from build123d import *

# Parameters (mm, degrees)
F0_R      = 20
F1_DEPTH  = 50
F3_R      = 10
F4_DEPTH  = 120
F6_R      = 10
F7_DEPTH  = 50
F8_R      = 2.533674
F9_DEPTH  = 101
F10_DEPTH = 101


with BuildPart() as f1:
    # F0 (on Front) → F1 (new body, symmetric)
    with BuildSketch(Plane.XZ):
        Circle(F0_R)
    extrude(amount=F1_DEPTH, both=True)

    # F3 (on offset) → F4 (cut)
    with BuildSketch(Plane.XZ.offset(60)):
        Circle(F3_R)
    extrude(amount=-F4_DEPTH, mode=Mode.SUBTRACT)

    # F6 (on offset) → F7 (cut, symmetric)
    with BuildSketch(Plane.YZ.offset(30)):
        Circle(F6_R)
    extrude(amount=F7_DEPTH, both=True, mode=Mode.SUBTRACT)

    # F8 (on face) → F9 (cut)
    with BuildSketch(Plane.XZ.offset(50)):
        with Locations((5.240558, 14.022033)):
            Circle(F8_R)
    extrude(amount=-F9_DEPTH, mode=Mode.SUBTRACT)

    # F8 (on face) → F10 (cut)
    with BuildSketch(Plane.XZ.offset(50)):
        with Locations((-5.240558, 14.022033)):
            Circle(F8_R)
        with Locations((-5.240558, -14.022033)):
            Circle(F8_R)
        with Locations((5.240558, -14.022033)):
            Circle(F8_R)
    extrude(amount=-F10_DEPTH, mode=Mode.SUBTRACT)


solid = f1.part
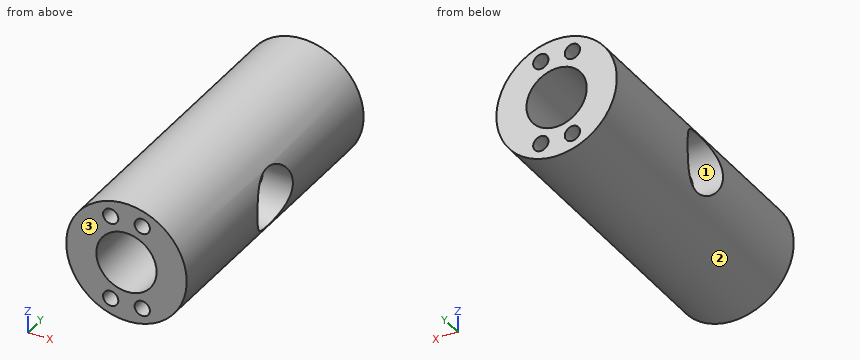
Design review of the part built by this model. Coordinates are the model's own, in mm. Face numbers are marked on the shaded views. Round coordinates to 2 decimals unless told otherwise and drop trailing zeros. Write each loop counter-clockwise with the first axis right and the second up, starting at its lowest first coordinate (ties: lowest second). Pieces come first, ordered by that corner, then holes. Notation, with made-up numbers: (2, 80.5) - (45, 80.5) arc R19 ccw to (45, 109.5) - close; hole circle Ø11 at (-24, 69). An arc over 180 degrees is marked (long way). Use a Markdown table: item, result. Add a question column.
1. We need section A-A (y = 4). State the section outline as (x, z) points.
2. Wall thickness on probe 1 along Z at (x, y) = (3, -35.5) (3 decimals); probe 2 along Z at (x, y) = (-5, -10); probe 3 along X at (y, z) = (-27.5, -15.5): over which ranges is each line inside the solid? List them lowest first.
3. We need section C-C (x = -16). State the section outline as (y, z) points.
4. We need section B-B (z = -4.5). State the section outline as (x, y) points.
5. We need section D-D (z = 0). State the section outline as (x, y) points.
6. Mouldability with a two-part tool opening along Z and no side actions: class the marked faces 1, 2 and 3 as +Z half, -Z half, draft (parallel to the pull), parting line (faces both ways), or undercut.
7. Clearance check with flat-ended pins moving along their axes: pin 1 (6.5 mm diameter, centred on x = 5.24, z = 14.02, fed in from -Y); pin 2 (6 mm diameter, centred on x = -15.5, y = 6, fed in from -Z); pin 3 (1.5 mm diameter, centred on y = 31, z = 5.5, fed in from -X); pin 4 (10 mm diameter, centred on x = 6.5, y = -3, fed in from -Z). State where each tip first meets the part, or that it passes through.
Output:
| question | item | result |
|---|---|---|
| 1 | outline | (-17.78, -9.17) arc R20 ccw to (17.78, -9.17) - (4, -9.17) arc R10 cw to (-4, -9.17) - close; (-17.78, 9.17) - (-4, 9.17) arc R10 cw to (4, 9.17) - (17.78, 9.17) arc R20 ccw to start; hole circle Ø5.07 at (-5.24, -14.02); hole circle Ø5.07 at (-5.24, 14.02); hole circle Ø5.07 at (5.24, -14.02); hole circle Ø5.07 at (5.24, 14.02) |
| 2 | probe 1 | z = -19.774 to -15.205, -12.839 to -9.539, 9.539 to 12.839, 15.205 to 19.774 |
| 2 | probe 2 | z = -19.36 to -16.54, -11.5 to -8.66, 8.66 to 11.5, 16.54 to 19.36 |
| 2 | probe 3 | x = -12.64 to -7.3, -3.18 to 3.18, 7.3 to 12.64 |
| 3 | outline | (-50, -12) - (50, -12) - (50, 12) - (-50, 12) - close; hole circle Ø20 at (0, 0) |
| 4 | outline | (-19.49, -50) - (-8.93, -50) - (-8.93, -8.93) - (-19.49, -8.93) - close; (-19.49, 8.93) - (-8.93, 8.93) - (-8.93, 50) - (-19.49, 50) - close; (8.93, -50) - (19.49, -50) - (19.49, -8.93) - (8.93, -8.93) - close; (8.93, 8.93) - (19.49, 8.93) - (19.49, 50) - (8.93, 50) - close |
| 5 | outline | (-20, -50) - (-10, -50) - (-10, -10) - (-20, -10) - close; (-20, 10) - (-10, 10) - (-10, 50) - (-20, 50) - close; (10, -50) - (20, -50) - (20, -10) - (10, -10) - close; (10, 10) - (20, 10) - (20, 50) - (10, 50) - close |
| 6 | face 1 | undercut |
| 6 | face 2 | parting line |
| 6 | face 3 | draft |
| 7 | pin 1 | stops at y = -50 |
| 7 | pin 2 | stops at z = -15.61 |
| 7 | pin 3 | stops at x = -19.43 |
| 7 | pin 4 | stops at z = -19.94 |
